from build123d import *

# Parameters (mm, degrees)
F1_DEPTH = 9.525
F3_D     = 6.35


with BuildPart() as f1:
    # F0 (on Front) → F1 (new body)
    with BuildSketch(Plane.XZ):
        with BuildLine():
            Line((0, 175.99378), (0, 27.20622))
            ThreePointArc((0, 27.20622), (8.123369, 11.601373), (25.565484, 9.305075))
            Line((25.565484, 9.305075), (177.965484, 64.774139))
            ThreePointArc((177.965484, 64.774139), (187.054846, 71.748652), (190.5, 82.675283))
            Line((190.5, 82.675283), (190.5, 120.524717))
            ThreePointArc((190.5, 120.524717), (187.054846, 131.451348), (177.965484, 138.425861))
            Line((177.965484, 138.425861), (25.565484, 193.894925))
            ThreePointArc((25.565484, 193.894925), (8.123369, 191.598627), (0, 175.99378))
        make_face()
    extrude(amount=F1_DEPTH)

    # F3 (through all)
    with Locations(Plane.XZ.offset(9.525)):
        with Locations((19.602309, 177.8), (19.602309, 101.6), (19.602309, 25.4)):
            Hole(F3_D / 2)


solid = f1.part
Verification items for the finished model (mm, model axes). Give positions to 0.01 mm unless a question says otherwise; leave off trailing zeros. Write each loop counter-clockwise with the first axis right and the second up, starting at its lowest first coordinate (ties: lowest second). Pieces come first, ordered by that corner, then holes.
(1) Cross-section at A-A (y = -5). Enter the section's corners in (x, z) (3 decimals), plus the area to 3 significant figures.
(2) Mould release check, pull along X, two halves, no side actions. Record for faces 1 (the face through (20.016, -4.696, 28.548)), 2 (the face through (8.33, -4.7, 191.74)), 3 (the face through (186.961, -4.696, 71.616)): +X half, -X half, draft (parallel to the pull), parting line (faces both ways), or undercut.
(3) Material ranges on line 1 (Z direction, x = 183.5, y = -8.5); line 2 (Z direction, x = 76, y = -5.5); line 3 (X direction, y = -0.25, z = 130.5), recorded low to high.
(4) Cross-section at D-D (z = 52.5). Enter the section's corners in (x, y) (3 decimals).
(5) Cross-section at C-C (x = 89.5). Enter the section's corners in (y, z) (3 decimals).
(6) Gauge pin test, flat end, axial feed: pin 1 (3 mm diameter, centred on x = 33, y = -6.5, fed in from -Z). Record the tip position at first contact, or that the pin passes through.
(7) Cross-section at B-B (z = 101.6). Enter the section's corners in (x, y) (3 decimals).
Worked out:
1. outline: (0, 27.206) arc R19.05 ccw to (25.565, 9.305) - (177.965, 64.774) arc R19.05 ccw to (190.5, 82.675) - (190.5, 120.525) arc R19.05 ccw to (177.965, 138.426) - (25.565, 193.895) arc R19.05 ccw to (0, 175.994) - close; hole circle Ø6.35 at (19.602, 25.4); hole circle Ø6.35 at (19.602, 101.6); hole circle Ø6.35 at (19.602, 177.8)
1. area: 25,000 mm2
2. face 1: undercut
2. face 2: parting line
2. face 3: +X half
3. line 1: z = 67.92 to 135.28
3. line 2: z = 27.66 to 175.54
3. line 3: x = 0 to 187.68
4. outline: (0, -9.525) - (144.243, -9.525) - (144.243, 0) - (0, 0) - close
5. outline: (-9.525, 32.575) - (0, 32.575) - (0, 170.625) - (-9.525, 170.625) - close
6. pin 1: stops at z = 11.47
7. outline: (0, -9.525) - (16.427, -9.525) - (16.427, 0) - (0, 0) - close; (22.777, -9.525) - (190.5, -9.525) - (190.5, 0) - (22.777, 0) - close
